```python
from build123d import *

# Parameters (mm, degrees)
CYLINDER001_R                    = 2.6
CYLINDER001_DEPTH                = 9
CYLINDER001002001_R              = 2.6
CYLINDER001002001_DEPTH          = 9
CYLINDER001002001001_R           = 2.6
CYLINDER001002001001_DEPTH       = 9
CYLINDER001002001001001_R        = 2.6
CYLINDER001002001001001_DEPTH    = 9
CYLINDER001002001001001001_R     = 2.6
CYLINDER001002001001001001_DEPTH = 9
CYLINDER001002_R                 = 2.6
CYLINDER001002_DEPTH             = 9
CYLINDER001001_R                 = 2.6
CYLINDER001001_DEPTH             = 9
CYLINDER_R                       = 70
CYLINDER_DEPTH                   = 20
CYLINDER002_R                    = 75
CYLINDER002_DEPTH                = 11


with BuildPart() as pole1:
    # Cylinder001 → Cylinder001 (new body)
    with BuildSketch(Plane(origin=(70, 0, 0), x_dir=(1, 0, 0), z_dir=(0, 0, 1))):
        Circle(CYLINDER001_R)
    extrude(amount=CYLINDER001_DEPTH)


with BuildPart() as pole2:
    # Cylinder001002001 → Cylinder001002001 (new body)
    with BuildSketch(Plane(origin=(67.55, 18.2, 0), x_dir=(1, 0, 0), z_dir=(0, 0, 1))):
        Circle(CYLINDER001002001_R)
    extrude(amount=CYLINDER001002001_DEPTH)


with BuildPart() as pole003:
    # Cylinder001002001001 → Cylinder001002001001 (new body)
    with BuildSketch(Plane(origin=(60.62, 35, 0), x_dir=(1, 0, 0), z_dir=(0, 0, 1))):
        Circle(CYLINDER001002001001_R)
    extrude(amount=CYLINDER001002001001_DEPTH)


with BuildPart() as pole004:
    # Cylinder001002001001001 → Cylinder001002001001001 (new body)
    with BuildSketch(Plane(origin=(49.49, 49.49, 0), x_dir=(1, 0, 0), z_dir=(0, 0, 1))):
        Circle(CYLINDER001002001001001_R)
    extrude(amount=CYLINDER001002001001001_DEPTH)


with BuildPart() as pole005:
    # Cylinder001002001001001001 → Cylinder001002001001001001 (new body)
    with BuildSketch(Plane(origin=(35, 60.62, 0), x_dir=(1, 0, 0), z_dir=(0, 0, 1))):
        Circle(CYLINDER001002001001001001_R)
    extrude(amount=CYLINDER001002001001001001_DEPTH)


with BuildPart() as pole006:
    # Cylinder001002 → Cylinder001002 (new body)
    with BuildSketch(Plane(origin=(18.2, 67.55, 0), x_dir=(1, 0, 0), z_dir=(0, 0, 1))):
        Circle(CYLINDER001002_R)
    extrude(amount=CYLINDER001002_DEPTH)


with BuildPart() as fusion:
    # Cylinder001001 → Cylinder001001 (new body)
    with BuildSketch(Plane(origin=(0, 70, 0), x_dir=(1, 0, 0), z_dir=(0, 0, 1))):
        Circle(CYLINDER001001_R)
    extrude(amount=CYLINDER001001_DEPTH)

    # Fusion: union pole1, pole2, pole003, pole004, pole005, pole006
    add(pole1.part)
    add(pole2.part)
    add(pole003.part)
    add(pole004.part)
    add(pole005.part)
    add(pole006.part)


with BuildPart() as part_mirroring:
    # Part__Mirroring: instance of Fusion
    add(fusion.part.mirror(Plane(origin=(0, 0, 0), x_dir=(1, 0, 0), z_dir=(0, 1, 0))))


with BuildPart() as part_mirroring001:
    # Part__Mirroring001: instance of Part__Mirroring
    add(part_mirroring.part.mirror(Plane(origin=(0, 0, 0), x_dir=(0, -1, 0), z_dir=(1, 0, 0))))


with BuildPart() as part_mirroring002:
    # Part__Mirroring002: instance of Part__Mirroring001
    add(part_mirroring001.part.mirror(Plane(origin=(0, 0, 0), x_dir=(1, 0, 0), z_dir=(0, 1, 0))))


with BuildPart() as fusion001:
    # Fusion001 base: copy of Fusion
    add(fusion.part)

    # Fusion001: union Part__Mirroring, Part__Mirroring001, Part__Mirroring002
    add(part_mirroring.part)
    add(part_mirroring001.part)
    add(part_mirroring002.part)


with BuildPart() as cylinder:
    # Cylinder → Cylinder (new body)
    with BuildSketch(Plane.XY):
        Circle(CYLINDER_R)
    extrude(amount=CYLINDER_DEPTH)


with BuildPart() as cut001:
    # Cylinder002 → Cylinder002 (new body)
    with BuildSketch(Plane.XY):
        Circle(CYLINDER002_R)
    extrude(amount=CYLINDER002_DEPTH)

    # Cut: cut Cylinder
    add(cylinder.part, mode=Mode.SUBTRACT)

    # Cut001: cut Fusion001
    add(fusion001.part, mode=Mode.SUBTRACT)


solid = cut001.part
```
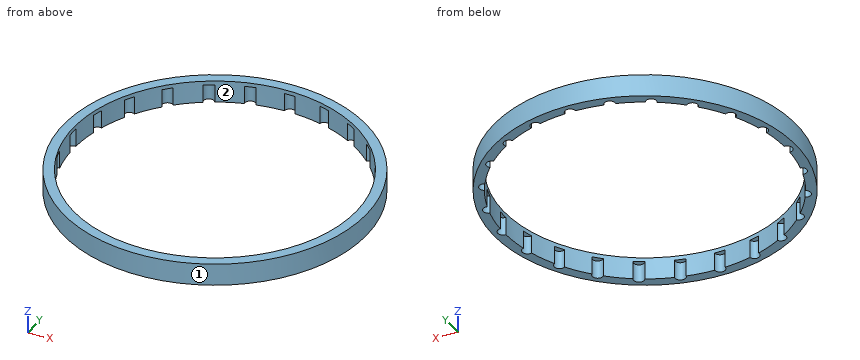
Input: part model. Units: mm. Frame: model coordinates. Face numbers are marked on the shaded views. Coordinates: 2 decimals unless noted, no trailing zeros. Loops run counter-clockwise (first coordinate to the right, second up) from the corner with the lowest first, then second, coordinate; pieces in that order, holes last.
Q1. Contact query for flat-ended pins moving along their axis: pin 1 (1.3 mm diameter, centred on x = 1.5, y = 71, fed in from -Z); pin 2 (1 mm diameter, centred on y = -4.5, z = 7, fed in from +X); pin 3 (4 mm diameter, centred on x = 7.5, z = 5, fed in from -Y). Output: stop coordinate, or through.
Results are:
pin 1: stops at z = 9
pin 2: stops at x = 74.89
pin 3: stops at y = -74.8
Q2. Section B-B, the plane x = -18.2. Return the cut outline in (y, z), and give its area (3 significant figures).
Results are:
outline: (-72.76, 0) - (-70.15, 0) - (-70.15, 9) - (-67.59, 9) - (-67.59, 11) - (-72.76, 11) - close; (67.59, 9) - (70.15, 9) - (70.15, 0) - (72.76, 0) - (72.76, 11) - (67.59, 11) - close
area: 67.6 mm2
Q3. Mould query, pull axis X, two halves, no side actions, for the marked faces 1 and 2. Classes: +X half, -X half, draft (parallel to the pull), parting line (faces both ways), or undercut.
Results are:
face 1: parting line
face 2: undercut
Q4. Section A-A, the plane y = 0. Return the cut outline in (x, z), and give its area (3 significant figures).
Results are:
outline: (-75, 0) - (-72.6, 0) - (-72.6, 9) - (-70, 9) - (-70, 11) - (-75, 11) - close; (70, 9) - (72.6, 9) - (72.6, 0) - (75, 0) - (75, 11) - (70, 11) - close
area: 63.2 mm2
Q5. Line query: line 1 along Y through (x, z) = (0, 6.5); line 2 along Y through (x, z) = (-39, 9); line 3 along X through (y, z) = (-51, 4.25). Output: solid intervals per line, ascending.
Results are:
line 1: y = -75 to -72.6, 72.6 to 75
line 2: y = -64.06 to -58.13, 58.13 to 64.06
line 3: x = -54.99 to -51.61, 51.61 to 54.99
